Geometry check sheet. Reference: the model listing, model coordinates, mm. Face numbers are marked on the shaded views. A direction names the side the tool comes from. Give positions to 0.01 mm unless a question says otherwise; leave off trailing zeros. Loops run counter-clockwise (first coordinate to the right, second up) from the corner with the lowest first, then second, coordinate; pieces in that order, holes last.
1. Tool access check on the marked faces 1, 2 and 3. Record the directions out of +Z, -Z, +X, -X, +Y, -Y that give a thin tool (end or side, any length) a straight path to the whole face; none if there is none.
2. Cross-section at B-B, the plane z = 9. Record the cut outline in (x, y) (3 decimals).
3. Cross-section at A-A, the plane y = 0. Record the cut outline in (x, z), plus the area to 3 significant figures.
4. Go/stop test with flat-tipped pins: pin 1 Ø12 at (x, z) = (13, 41.5) entering from -Y; pin 2 Ø18.5 at (x, y) = (9.5, -3) entering from +Z; pin 3 Ø14 at (x, z) = (9.5, -13) entering from -Y. Record where each tip stops, or that it passes through.
5. Cross-section at D-D, the plane y = 30. Record the cut outline in (x, z).
6. Cross-section at C-C, the plane x = 19.5. Record the cut outline in (y, z).
7. Release check for a two-part mould opening along Y. For the marked faces 4, 5 and 6 record: +Y half, -Y half, draft (parallel to the pull), parting line (faces both ways), or undercut.
8. Material ranges on L1, parallel to Z at x = 8.5, y = -1.5; L2, parallel to Z at x = 2.5, y = -31.5; L3, parallel to Z at x = 36.5, y = 18.5, recorded low to high.
from build123d import *

# Parameters (mm, degrees)
F1_R      = 50.8
F2_DEPTH  = 50.8
F4_R      = 4.445
F5_DEPTH  = 15.24
F6_DEPTH  = 12.7
F8_DEPTH  = 12.7
F9_DEPTH  = 25.4
F10_R     = 31.75
F10_R_2   = 22.86
F11_DEPTH = 63.5
F13_W     = 63.243523
F13_H     = 123.192005
F14_DEPTH = 127
F16_R     = 4.445
F17_DEPTH = 25.4


with BuildPart() as f2:
    # F1 (on offset) → F2 (new body)
    with BuildSketch(Plane.XY.offset(12.7)):
        Circle(F1_R)
    extrude(amount=-F2_DEPTH)

    # F4 (on offset) → F5 (cut)
    with BuildSketch(Plane.XZ.offset(50.8)):
        with Locations((0, -25.462054)):
            Circle(F4_R)
    extrude(amount=-F5_DEPTH, mode=Mode.SUBTRACT)

    # F4 (on offset) → F6 (cut)
    with BuildSketch(Plane.XZ.offset(50.8)):
        with Locations((0, -25.462054)):
            Circle(F4_R)
    extrude(amount=-F6_DEPTH, mode=Mode.SUBTRACT)

    # F7 (on Right) → F8 (cut)
    with BuildSketch(Plane.YZ):
        Polygon((4.88417, -30.198015), (4.88417, 0), (-4.341668, 0), (-38.032606, 0), (-38.032606, -30.198015), align=None)
    extrude(amount=F8_DEPTH, mode=Mode.SUBTRACT)

    # F7 (on Right) → F9 (cut)
    with BuildSketch(Plane.YZ):
        Polygon((4.88417, -30.198015), (4.88417, 0), (-4.341668, 0), (-38.032606, 0), (-38.032606, -30.198015), align=None)
    extrude(amount=-F9_DEPTH, mode=Mode.SUBTRACT)

    # F10 (on offset) → F11 (join)
    with BuildSketch(Plane.XY.offset(12.7)):
        Circle(F10_R)
        Circle(F10_R_2, mode=Mode.SUBTRACT)
    extrude(amount=F11_DEPTH)

    # F13 (on offset) → F14 (cut)
    with BuildSketch(Plane.XY.offset(76.2)):
        with Locations((-31.621761, -5.643372)):
            Rectangle(F13_W, F13_H)
    extrude(amount=-F14_DEPTH, mode=Mode.SUBTRACT)

    # F16 (on offset) → F17 (cut)
    with BuildSketch(Plane.XY.offset(19.05)):
        with Locations((0, -27.301347)):
            Circle(F16_R)
    extrude(amount=-F17_DEPTH, mode=Mode.SUBTRACT)


solid = f2.part
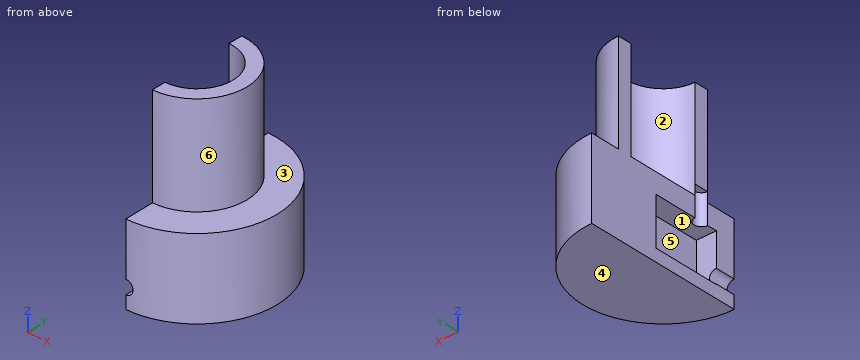
Result:
1. face 1: -X
1. face 2: +Z, -X
1. face 3: +Z, +X
2. outline: (0, -50.8) arc R50.8 ccw to (0, 50.8) - (0, -22.856) arc R4.445 cw to (0, -31.746) - close
3. outline: (0, -38.1) - (50.8, -38.1) - (50.8, 12.7) - (31.75, 12.7) - (31.75, 76.2) - (22.86, 76.2) - (22.86, 12.7) - (0, 12.7) - (0, 0) - (12.7, 0) - (12.7, -30.2) - (0, -30.2) - close
3. area: 2,760 mm2
4. pin 1: stops at y = -30.97
4. pin 2: stops at z = 12.7
4. pin 3: stops at y = -50.74
5. outline: (0, -38.1) - (41, -38.1) - (41, 12.7) - (10.4, 12.7) - (10.4, 76.2) - (0, 76.2) - close
6. outline: (-46.91, -38.1) - (46.91, -38.1) - (46.91, 12.7) - (25.06, 12.7) - (25.06, 76.2) - (11.93, 76.2) - (11.93, 12.7) - (-11.93, 12.7) - (-11.93, 76.2) - (-25.06, 76.2) - (-25.06, 12.7) - (-46.91, 12.7) - close
7. face 4: draft
7. face 5: undercut
7. face 6: parting line
8. L1: z = -38.1 to -30.2, 0 to 12.7
8. L2: z = -38.1 to -30.2, 0 to 76.2
8. L3: z = -38.1 to 12.7
